from build123d import *

# Parameters (mm, degrees)
BOSS_EXTRUDE1_DEPTH = 70
SKETCH2_W           = 50
SKETCH2_H           = 10
BOSS_EXTRUDE2_DEPTH = 12
BOSS_EXTRUDE3_DEPTH = 25
BOSS_EXTRUDE4_DEPTH = 25


with BuildPart() as part:
    # Sketch1 → Boss-Extrude1 (new body)
    with BuildSketch(Plane(origin=(0, 0, 0), x_dir=(0, 0, -1), z_dir=(1, 0, 0))):
        Polygon((0, 0), (0, 56.641016151), (-15, 56.641016151), (-75, 22), (-75, 0), (-50, 0), (-50, 11), (-15, 11), (-15, 0), align=None)
    extrude(amount=BOSS_EXTRUDE1_DEPTH)

    # Sketch2 → Boss-Extrude2 (add)
    with BuildSketch(Plane.XY.offset(75)):
        with Locations((35, 11)):
            Rectangle(SKETCH2_W, SKETCH2_H)
    extrude(amount=BOSS_EXTRUDE2_DEPTH)

    # Sketch3 → Boss-Extrude3 (add, symmetric)
    with BuildSketch(Plane(origin=(35, 0, 0), x_dir=(0, 0, -1), z_dir=(1, 0, 0))):
        with BuildLine():
            Line((-15, 75), (0, 75))
            Line((0, 75), (0, 56.641016151))
            Line((0, 56.641016151), (-15, 56.641016151))
            Line((-15, 56.641016151), (-54.974141253, 33.561934939))
            ThreePointArc((-54.974141253, 33.561934939), (-43.788214624, 62.771184684), (-15, 75))
        make_face()
    extrude(amount=BOSS_EXTRUDE3_DEPTH, both=True)

    # Sketch4 → Boss-Extrude4 (add)
    with BuildSketch(Plane(origin=(35, 0, 0), x_dir=(0, 0, -1), z_dir=(1, 0, 0))):
        Polygon((0, 75), (0, 85), (-8, 85), (-15, 75), align=None)
    extrude(amount=-BOSS_EXTRUDE4_DEPTH)


solid = part.part
Build history of the part. All positions in model axes, mm. A direction names the side the tool comes from. Coordinates: 2 decimals unless noted, no trailing zeros. Order: outer loops, then holes, each group sorted by start corner. A loop starts at its lowest first (then second) coordinate and runs counter-clockwise, first axis right, second up. Notation, with made-up numbers: (30.5, 65.5) -> (68.5, 65.5) arc R29 ccw to (68.5, 87.5) -> close; hole circle Ø5 at (1.5, -25.75). An arc over 180 degrees is marked (long way). One line per item, written item: value.
(1) Slice it at C-C, the plane z = 41. List the corners of the cut face in (x, y), plus the area to 3 significant figures.
Checked values:
outline: (0, 11) -> (70, 11) -> (70, 41.63) -> (60, 41.63) -> (60, 65.4) -> (10, 65.4) -> (10, 41.63) -> (0, 41.63) -> close
area: 3,330 mm2
(2) Mould opens along Z. For faces 6 (the flat face through (5, 56.641, 7)), 7 (the flat face through (35, 11, 33)), 8 (the cylindrical face through (35.35, 62.446, 44.099)) say: pulls with the +Z half, pulls with the -Z half, needs draft (parallel to the pull), parting line crosses it, or undercut.
Checked values:
face 6: needs draft
face 7: undercut
face 8: pulls with the +Z half
(3) Slice it at B-B, the plane y = 43. List the corners of the cut face in (x, z), plus the area to 3 significant figures.
Checked values:
outline: (0, 0) -> (70, 0) -> (70, 38.63) -> (60, 38.63) -> (60, 54.19) -> (10, 54.19) -> (10, 38.63) -> (0, 38.63) -> close
area: 3,480 mm2
(4) Probe line 1 (Z direction, x = 26.5, y = 9.5); line 2 (Z direction, x = 63.5, y = 15); line 3 (Y direction, x = 13, z = 79.5). List the from-to ranges inside material, lowest first. Write a range as [from, to].
Checked values:
line 1: [0, 15], [50, 87]
line 2: [0, 75]
line 3: [6, 16]
(5) Drop flat-ended pins along their axis: pin 1 Ø6 at (x, z) = (45.5, 84) entering from -Y; pin 2 Ø3 at (y, z) = (12.5, 81) entering from -X; pin 3 Ø9.5 at (x, z) = (32, 82.5) entering from +Y. Give the stop position or say it passes through.
Checked values:
pin 1: y = 6
pin 2: x = 10
pin 3: y = 16
(6) Slice it at D-D, the plane x = 13. List the corners of the cut face in (y, z), plus the area to 3 significant figures.
Checked values:
outline: (0, 0) -> (85, 0) -> (85, 8) -> (75, 15) arc R40 ccw to (33.56, 54.97) -> (22, 75) -> (16, 75) -> (16, 87) -> (6, 87) -> (6, 75) -> (0, 75) -> (0, 50) -> (11, 50) -> (11, 15) -> (0, 15) -> close
area: 4,190 mm2
(7) Slice it at A-A, the plane x = 65. List the corners of the cut face in (y, z), plus the area to 3 significant figures.
Checked values:
outline: (0, 0) -> (56.64, 0) -> (56.64, 15) -> (22, 75) -> (0, 75) -> (0, 50) -> (11, 50) -> (11, 15) -> (0, 15) -> close
area: 2,820 mm2
(8) Tool access for faces 1 (the flat face through (35, 16, 81)), 2 (the flat face through (10, 11, 81)), 3 (the flat face through (35, 6, 81)), 4 (the flat face through (35, 5, 50)), 5 (the flat face through (48, 75, 8)): list every direction of +Z, -Z, +X, -X, +Y, -Y with a clear straight run to the whole face (end or side of a thin tool).
Checked values:
face 1: +Z, +X, -X, +Y
face 2: +Z, -X, +Y, -Y
face 3: +Z, +X, -X, -Y
face 4: +X, -X, -Y
face 5: +Z, -Z, +X, +Y
